from build123d import *

# Parameters (mm, degrees)
SKETCH1_W           = 279.4
SKETCH1_H           = 76.2
BOSS_EXTRUDE1_DEPTH = 5.08
SKETCH2_W           = 254
SKETCH2_H           = 38.1
CUT_EXTRUDE1_DEPTH  = 145.891360681
FILLET1_R           = 12.7
FILLET2_R           = 12.7
SKETCH4_W           = 203.2
SKETCH4_H           = 12.7
CUT_EXTRUDE2_DEPTH  = 145.891360681
SKETCH5_W           = 25.4
SKETCH5_H           = 5.08
BOSS_EXTRUDE2_DEPTH = 5.08
FILLET3_R           = 5.08
CUT_EXTRUDE4_DEPTH  = 145.891360681


with BuildPart() as part:
    # Sketch1 → Boss-Extrude1 (new body)
    with BuildSketch(Plane(origin=(0, 0, 0), x_dir=(1, 0, 0), z_dir=(0, 1, 0))):
        Rectangle(SKETCH1_W, SKETCH1_H)
    extrude(amount=BOSS_EXTRUDE1_DEPTH)

    # Sketch2 → Cut-Extrude1 (cut, through all)
    with BuildSketch(Plane(origin=(0, 5.08, 0), x_dir=(1, 0, 0), z_dir=(0, 1, 0))):
        with Locations((0, -6.35)):
            Rectangle(SKETCH2_W, SKETCH2_H)
    extrude(amount=-CUT_EXTRUDE1_DEPTH, mode=Mode.SUBTRACT)

    # Fillet1
    fillet1_edges = [part.edges().sort_by_distance(p)[0] for p in [
        (-139.7, 2.54, -38.1),
        (139.7, 2.54, -38.1),
    ]]
    fillet(fillet1_edges, radius=FILLET1_R)

    # Fillet2
    fillet2_edges = [part.edges().sort_by_distance(p)[0] for p in [
        (139.7, 2.54, 38.1),
        (-139.7, 2.54, 38.1),
    ]]
    fillet(fillet2_edges, radius=FILLET2_R)

    # Sketch4 → Cut-Extrude2 (cut, through all)
    with BuildSketch(Plane(origin=(0, 5.08, 0), x_dir=(1, 0, 0), z_dir=(0, 1, 0))):
        with Locations((0, -31.75)):
            Rectangle(SKETCH4_W, SKETCH4_H)
    extrude(amount=-CUT_EXTRUDE2_DEPTH, mode=Mode.SUBTRACT)

    # Sketch5 → Boss-Extrude2 (add)
    with BuildSketch(Plane.XY.offset(-12.7)):
        with Locations((0, 2.54)):
            Rectangle(SKETCH5_W, SKETCH5_H)
    extrude(amount=BOSS_EXTRUDE2_DEPTH)

    # Fillet3
    fillet3_edges = [part.edges().sort_by_distance(p)[0] for p in [
        (-12.7, 2.54, -7.62),
        (12.7, 2.54, -7.62),
    ]]
    fillet(fillet3_edges, radius=FILLET3_R - 0.0001)  # a hair under: the kernel refuses the full size

    # Sketch6 → Cut-Extrude4 (cut, through all)
    with BuildSketch(Plane(origin=(0, 5.08, 0), x_dir=(1, 0, 0), z_dir=(0, 1, 0))):
        with BuildLine():
            Line((-4.445, 15.24), (-4.445, 25.4))
            ThreePointArc((-4.445, 25.4), (0, 29.845), (4.445, 25.4))
            Line((4.445, 25.4), (4.445, 15.24))
            ThreePointArc((4.445, 15.24), (0, 10.795), (-4.445, 15.24))
        make_face()
    extrude(amount=-CUT_EXTRUDE4_DEPTH, mode=Mode.SUBTRACT)


solid = part.part
Model file for the job. Use its own axes, mm. A direction names the side the tool comes from. Give positions to 0.01 mm unless a question says otherwise; leave off trailing zeros. Order: outer loops, then holes, each group sorted by start corner. A loop starts at its lowest first (then second) coordinate and runs counter-clockwise, first axis right, second up. Notation, with made-up numbers: M 78.5,9.5 L 96.5,9.5 A14 cw 96.5,28.5 Z; hole C -29,56 d4. An arc over 180 degrees is marked long. Put each result on its own line as item: value. Start each with the question number.
(1) Pin check, flat tips, straight feed: pin 1 Ø1.5 at (y, z) = (2, 33) entering from +X; pin 2 Ø2 at (x, y) = (63, 3) entering from +Z; pin 3 Ø2 at (x, y) = (-9, 3.5) entering from +Z. Stop position of each tip, or through.
(2) Pull direction Z, two halves, no side cores. Call faces 1 (the face through (-127, 3, 7)), 2 (the face through (-101.6, 3, 32)), 3 (the face through (-11.251, 2.576, -9.148)): released by +Z, released by -Z, zero draft, split by the parting line, or undercut.
(3) Band-saw the part on D-D on x = -98. Give the cut face in (y, z).
(4) Band-saw the part on A-A on x = 0. Give the cut face in (y, z) (3 decimals), then the cut area to 3 significant figures.
(5) Drill centre lines: L1, parallel to X at y = 4.65, z = -3.5; L2, parallel to Z at x = -123, y = 0.3; L3, parallel to X at y = 4.8, z = -22 (3 decimals). Where is each one in solid material? Low to high. Write a range as [from, to].
(6) Band-saw the part on C-C on z = 28.5. Give the cut face in (x, y).
(7) Tool access for faces 4 (the face through (101.6, 3, 32)), 5 (the face through (-1, 5.08, -9)), 6 (the face through (4.445, 3, -20)): list every direction of +Z, -Z, +X, -X, +Y, -Y with a clear straight run to the whole face (end or side of a thin tool).
Results below:
1. pin 1: stops at x = 137.69
1. pin 2: stops at z = -12.7
1. pin 3: stops at z = -7.63
2. face 1: undercut
2. face 2: zero draft
2. face 3: released by +Z
3. outline: M 0,-38.1 L 5.08,-38.1 L 5.08,-12.7 L 0,-12.7 Z
4. outline: M 0,-38.1 L 5.08,-38.1 L 5.08,-29.845 L 0,-29.845 Z; M 0,-10.795 L 5.08,-10.795 L 5.08,-7.62 L 0,-7.62 Z
4. area: 58.1 mm2
5. L1: x = [-139.7, -127], [127, 139.7]
5. L2: z = [-38.1, -12.7], [25.4, 38.1]
5. L3: x = [-139.7, -4.445], [4.445, 139.7]
6. outline: M -139.32,0 L -101.6,0 L -101.6,5.08 L -139.32,5.08 Z; M 101.6,0 L 139.32,0 L 139.32,5.08 L 101.6,5.08 Z
7. face 4: +Z, +Y, -Y
7. face 5: +Z, -Z, +X, -X, +Y
7. face 6: +Y, -Y
